from build123d import *

# Parameters (mm, degrees)
CROQUIS2_W              = 37.5
CROQUIS2_H              = 32
SALIENTE_EXTRUIR1_DEPTH = 10
CROQUIS7_R              = 1.65
CUT_EXTRUDE_1_DEPTH     = 10
CROQUIS13_R             = 1.65
CUT_EXTRUDE_3_DEPTH     = 6
CUT_EXTRUDE_START       = -6
CUT_EXTRUDE_4_DEPTH     = 6
SKETCH_7_W              = 24
SKETCH_7_H              = 10
CUT_EXTRUDE_5_DEPTH     = 12


with BuildPart() as part:
    # Croquis2 → Saliente-Extruir1 (new body)
    with BuildSketch(Plane(origin=(0, 0, 0), x_dir=(1, 0, 0), z_dir=(0, 1, 0))):
        with Locations((17.25, 7.5)):
            Rectangle(CROQUIS2_W, CROQUIS2_H)
    extrude(amount=SALIENTE_EXTRUIR1_DEPTH)

    # Croquis7 → 切除-拉伸1 (cut)
    with BuildSketch(Plane.XZ):
        with Locations(Location((3.5, -18.5, 0), (0, 0, 270))):
            Circle(CROQUIS7_R)
        with Locations(Location((16, -18.5, 0), (0, 0, 270))):
            Circle(CROQUIS7_R)
        with Locations(Location((3.5, 3.5, 0), (0, 0, 270))):
            Circle(CROQUIS7_R)
        with Locations(Location((16, 3.5, 0), (0, 0, 270))):
            Circle(CROQUIS7_R)
    extrude(amount=-CUT_EXTRUDE_1_DEPTH, mode=Mode.SUBTRACT)

    # Croquis13 → 切除-拉伸3 (cut)
    with BuildSketch(Plane.XY.offset(8.5)):
        with Locations((29.25, 5)):
            Circle(CROQUIS13_R)
    extrude(amount=-CUT_EXTRUDE_3_DEPTH, mode=Mode.SUBTRACT)

    # 草图6 → 切除-拉伸4 (cut)
    with BuildSketch(Plane(origin=(0, 0, -23.5), x_dir=(-1, 0, 0), z_dir=(0, 0, -1)).offset(CUT_EXTRUDE_START)):
        with BuildLine():
            ThreePointArc((-27.6, 5), (-28.083273811, 6.166726189), (-29.25, 6.65))
            Line((-29.25, 6.65), (-29.25, 3.35))
            ThreePointArc((-29.25, 3.35), (-28.083273811, 3.833273811), (-27.6, 5))
        make_face()
        with BuildLine():
            Line((-29.25, 3.35), (-29.25, 6.65))
            ThreePointArc((-29.25, 6.65), (-30.9, 5), (-29.25, 3.35))
        make_face()
    extrude(amount=CUT_EXTRUDE_4_DEPTH, mode=Mode.SUBTRACT)

    # 草图7 → 切除-拉伸5 (cut)
    with BuildSketch(Plane(origin=(36, 0, 0), x_dir=(0, 0, -1), z_dir=(1, 0, 0))):
        with Locations((7.5, 5)):
            Rectangle(SKETCH_7_W, SKETCH_7_H)
    extrude(amount=-CUT_EXTRUDE_5_DEPTH, mode=Mode.SUBTRACT)


solid = part.part
Geometry: final body of the model. Coordinates: model frame, mm. A direction names the side the tool comes from. Give positions to 0.01 mm unless a question says otherwise; leave off trailing zeros. Order: outer loops, then holes, each group sorted by start corner. A loop starts at its lowest first (then second) coordinate and runs counter-clockwise, first axis right, second up. Notation, with made-up numbers: (-12, -7) -> (-7, -7) arc R6 cw to (-7, 0) -> close; hole circle Ø6 at (67.5, 81). An arc over 180 degrees is marked (long way). Answer as a JSON object with one key per item and string values.
Q1. First-contact query: pin 1 (1.5 mm diameter, centred on y = 8.5, z = -13.5, fed in from +X). Flat tip, straight axial feed; report the tip coordinate or a pass-through.
Entries:
{"pin 1": "stops at x = 24"}
Q2. Material intervals for probe 1 along X at (y, z) = (6, -18.5); probe 2 along Y at (x, z) = (29.25, 7.4); probe 3 along Z at (x, y) = (28, 3.75), sorted ascending.
Entries:
{"probe 1": "x = -1.5 to 1.85, 5.15 to 14.35, 17.65 to 24", "probe 2": "y = 0 to 3.35, 6.65 to 10", "probe 3": "z = -23.5 to -19.5, 4.5 to 8.5"}
Q3. Draft query along X for faces 1 (the cylindrical face through (3.57, 4.93, 5.15)), 2 (the flat face through (-1.5, 5, -7)), 3 (the flat face through (13, 0, -8)), 4 (the cylindrical face through (16.496, 4.93, -20.074)). Return one class per face: released by +X, released by -X, zero draft, split by the parting line, or undercut.
Entries:
{"face 1": "undercut", "face 2": "released by -X", "face 3": "zero draft", "face 4": "undercut"}
Q4. Section C-C (x = 32.5). Output: boundary loops of the cut face in (y, z).
Entries:
{"outline": "(0, -23.5) -> (10, -23.5) -> (10, -19.5) -> (0, -19.5) -> close; (0, 4.5) -> (10, 4.5) -> (10, 8.5) -> (0, 8.5) -> close"}
Q5. Section D-D (x = 3.5). Output: boundary loops of the cut face in (y, z), plus the area to 3 significant figures.
Entries:
{"outline": "(0, -23.5) -> (10, -23.5) -> (10, -20.15) -> (0, -20.15) -> close; (0, -16.85) -> (10, -16.85) -> (10, 1.85) -> (0, 1.85) -> close; (0, 5.15) -> (10, 5.15) -> (10, 8.5) -> (0, 8.5) -> close", "area": "254 mm^2"}
Q6. Section B-B (y = 4.25). Output: boundary loops of the cut face in (x, z), plus the area to 3 significant figures.
Entries:
{"outline": "(-1.5, -23.5) -> (27.78, -23.5) -> (27.78, -19.5) -> (24, -19.5) -> (24, 4.5) -> (27.78, 4.5) -> (27.78, 8.5) -> (-1.5, 8.5) -> close; (30.72, -23.5) -> (36, -23.5) -> (36, -19.5) -> (30.72, -19.5) -> close; (30.72, 4.5) -> (36, 4.5) -> (36, 8.5) -> (30.72, 8.5) -> close; hole circle Ø3.3 at (3.5, -18.5); hole circle Ø3.3 at (3.5, 3.5); hole circle Ø3.3 at (16, -18.5); hole circle Ø3.3 at (16, 3.5)", "area": "854 mm^2"}
Q7. Section A-A (z = -18.5). Output: boundary loops of the cut face in (x, y).
Entries:
{"outline": "(-1.5, 0) -> (1.85, 0) -> (1.85, 10) -> (-1.5, 10) -> close; (5.15, 0) -> (14.35, 0) -> (14.35, 10) -> (5.15, 10) -> close; (17.65, 0) -> (24, 0) -> (24, 10) -> (17.65, 10) -> close"}
Q8. Access query for faces 5 (the flat face through (24, 5, -7)), 6 (the cylindrical face through (17.115, 4.93, 4.716)). Directions: +Z, -Z, +X, -X, +Y, -Y. A direction counts if a zero-diameter tool reaches every point of the face in a straight line with its end or side. Return the directions, or none.
Entries:
{"face 5": "+X, +Y, -Y", "face 6": "+Y, -Y"}
